Verification items for the finished model (mm, model axes). Face numbers are marked on the shaded views. A direction names the side the tool comes from. Round coordinates to 2 decimals unless told otherwise and drop trailing zeros. Order: outer loops, then holes, each group sorted by start corner. A loop starts at its lowest first (then second) coordinate and runs counter-clockwise, first axis right, second up. Notation, with made-up numbers: (55.25, -32) -> (76.25, -32) arc R10 ccw to (76.25, -13) -> close; hole circle Ø3 at (15.5, 34.5). An arc over 180 degrees is marked (long way). Put each result on its own line as item: value.
```python
from build123d import *

# Parameters (mm, degrees)
SKETCH1_W           = 18
SKETCH1_H           = 33
BOSS_EXTRUDE1_DEPTH = 46
CUT_EXTRUDE1_DEPTH  = 8
SKETCH4_R           = 6.5
CUT_EXTRUDE2_DEPTH  = 10
FILLET3_R           = 5
FILLET4_R           = 7
CUT_EXTRUDE3_DEPTH  = 8


with BuildPart() as part:
    # Sketch1 → Boss-Extrude1 (new body)
    with BuildSketch(Plane(origin=(0, 0, 0), x_dir=(1, 0, 0), z_dir=(0, 1, 0))):
        Rectangle(SKETCH1_W, SKETCH1_H)
    extrude(amount=BOSS_EXTRUDE1_DEPTH)

    # Boss-Extrude2 cone 1 section (through the dimple's axis) → Boss-Extrude2 (revolve)
    with BuildSketch(Plane(origin=(0, 46, 0), x_dir=(0, 0, -1), z_dir=(1, 0, 0))):
        Polygon((0, 0), (7, 0), (0, 39.698972737), align=None)
    revolve(axis=Axis((0, 46, 0), (0, 1, 0)))

    # Sketch3 → Cut-Extrude1 (cut)
    with BuildSketch(Plane.ZY.offset(9)):
        with BuildLine():
            Line((-16.5, 0), (16.5, 0))
            Line((16.5, 0), (16.5, 20))
            ThreePointArc((16.5, 20), (0, 36.5), (-16.5, 20))
            Line((-16.5, 20), (-16.5, 0))
        make_face()
    extrude(amount=-CUT_EXTRUDE1_DEPTH, mode=Mode.SUBTRACT)

    # Sketch4 → Cut-Extrude2 (cut)
    with BuildSketch(Plane.ZY.offset(1)):
        with Locations((0, 20)):
            Circle(SKETCH4_R)
    extrude(amount=-CUT_EXTRUDE2_DEPTH, mode=Mode.SUBTRACT)

    # Fillet3
    fillet3_edges = [part.edges().sort_by_distance(p)[0] for p in [
        (4, 0, 16.5),
        (4, 0, -16.5),
    ]]
    fillet(fillet3_edges, radius=FILLET3_R)

    # Fillet4
    fillet4_edges = [part.edges().sort_by_distance(p)[0] for p in [
        (0, 46, 16.5),
        (0, 46, -16.5),
    ]]
    fillet(fillet4_edges, radius=FILLET4_R)

    # Sketch6 → Cut-Extrude3 (cut)
    with BuildSketch(Plane.ZY.offset(9)):
        with BuildLine():
            Line((-16.5, 20), (16.5, 20))
            Line((16.5, 20), (16.5, 28.185352772))
            ThreePointArc((16.5, 28.185352772), (0, 41.092676386), (-16.5, 28.185352772))
            Line((-16.5, 28.185352772), (-16.5, 20))
        make_face()
    extrude(amount=-CUT_EXTRUDE3_DEPTH, mode=Mode.SUBTRACT)


solid = part.part
```
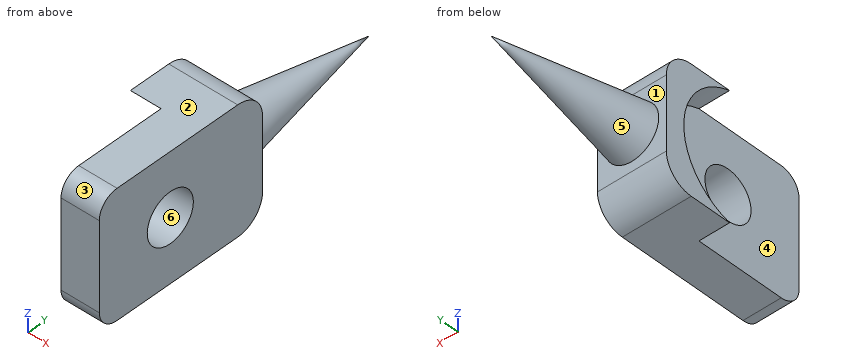
Item 1: Sectioned sample at D-D, the plane y = 75. Record the boundary of the cut face in (x, z).
Geometry check:
outline: circle Ø3.77 at (0, 0)
Item 2: Sectioned sample at C-C, the plane z = 10.5. Record the boundary of the cut face in (x, y), then the cut area to 3 significant figures.
Geometry check:
outline: (-9, 37.46) -> (-1, 37.46) -> (-1, 0) -> (9, 0) -> (9, 45.93) -> (-9, 45.93) -> close
area: 527 mm2
Item 3: Sectioned sample at A-A, the plane y = 20. Record the boundary of the cut face in (x, z).
Geometry check:
outline: (-1, -16.5) -> (9, -16.5) -> (9, -6.5) -> (-1, -6.5) -> close; (-1, 6.5) -> (9, 6.5) -> (9, 16.5) -> (-1, 16.5) -> close
Item 4: Depth check by flat-ended pin: pin 1 Ø8 at (x, y) = (2.5, 72) entering from -Z; pin 2 Ø6 at (x, y) = (-5.5, 74) entering from -Z; pin 3 Ø6 at (x, y) = (-1, 64.5) entering from -Z. Enter the tip coordinate at first touch or a pass-through.
Geometry check:
pin 1: z = -2.99
pin 2: through
pin 3: z = -4.24
Item 5: Sectioned sample at B-B, the plane y = 6. Record the boundary of the cut face in (x, z).
Geometry check:
outline: (-1, -16.5) -> (9, -16.5) -> (9, 16.5) -> (-1, 16.5) -> close
Item 6: Material ranges on line 1 along Z through (x, y) = (6.75, 20); line 2 along X through (y, z) = (19, 11); line 3 along Y through (x, z) = (4, -7), recorded low to high.
Geometry check:
line 1: -16.5 to -6.5, 6.5 to 16.5
line 2: -1 to 9
line 3: 0 to 46
Item 7: Tool access check on the marked faces 1 and 2. Record the directions out of +Z, -Z, +X, -X, +Y, -Y that give a thin tool (end or side, any length) a straight path to the whole face; none if there is none.
Geometry check:
face 1: +Y
face 2: +Z, +X, -X, +Y, -Y
Item 8: Release check for a two-part mould opening along Y. For the marked faces 3, 4, 5 and 6 record: pulls with the +Y half, pulls with the -Y half, needs draft (parallel to the pull), parting line crosses it, or undercut.
Geometry check:
face 3: pulls with the -Y half
face 4: needs draft
face 5: pulls with the +Y half
face 6: undercut
